Here's how the part is built. I have some questions about the finished solid (model axes, mm). A direction names the side the tool comes from. Give positions to 0.01 mm unless a question says otherwise; leave off trailing zeros. Loops run counter-clockwise (first coordinate to the right, second up) from the corner with the lowest first, then second, coordinate; pieces in that order, holes last. Notation, with made-up numbers: (-18.75, -27) -> (-8.75, -27) arc R22 ccw to (-8.75, -14) -> close; hole circle Ø4 at (10, -3). An arc over 180 degrees is marked (long way). Answer in a Markdown table with one row per item. Add a question column.
Item 1: If I drill on line 1 (Z direction, x = 0, y = -0.5); line 2 (X direction, y = -3.5, z = -223); line 3 (X direction, y = -0.5, z = -308.5), over which ranges is the centre line in solid material (lowest first)?
Item 2: For P1, Ø1.5, axis at x = 2.5, z = -62.5, coming from the +Y side; P2, Ø3.5, axis at x = 0, z = -308.5, coming from the -Y side; P3, Ø3, axis at x = -1, z = -114, coming from the -Y side, each with a flat end and sliding along its axis, tell me the tip position at first contact or that it passes through.
Item 3: If we section it at A-A (y = -8.75): Write out the boundary of the cut face in (x, z), then the cut area to 3 significant figures.
Item 4: Which directions (+Z, -Z, +X, -X, +Y, -Y) give clear straight access to the entire face, cutting with the end or side of a thin tool? Please do faces 1 (the face through (5.016, -7, -175)), 2 (the face through (1, -1, 0)).
Item 5: If we section it at C-C (x = -0.25): Write out the boundary of the cut face in (y, z), then the cut area to 3 significant figures.
Item 6: We'd pull the mould along X, two halves only. Please class faces 3 (the face through (0, 0, -175)), 4 (the face through (0, -1.588, -175)), 5 (the face through (6.604, -6, -175)): released by +X, released by -X, zero draft, split by the parting line, or undercut.
Item 7: If we section it at B-B (z = -218): Write out the boundary of the cut face in (x, y), then the cut area to 4 significant figures.
```python
from build123d import *

# Parameters (mm, degrees)
BOSS_EXTRUDE1_DEPTH  = 355
M4_CLEARANCE_HOLE2_D = 4.5


with BuildPart() as part:
    # Sketch1 → Boss-Extrude1 (new body)
    with BuildSketch(Plane.XY):
        Polygon((-6.604, 0), (6.604, 0), (6.604, -12.7), (5.0165, -12.7), (5.0165, -1.5875), (-5.0165, -1.5875), (-5.0165, -12.7), (-6.604, -12.7), align=None)
    extrude(amount=-BOSS_EXTRUDE1_DEPTH)

    # M4 Clearance Hole2 (through all)
    with Locations(Plane(origin=(0, 0, 0), x_dir=(1, 0, 0), z_dir=(0, 1, 0))):
        with Locations((0, 288.5), (0, 7), (0, 348.5), (0, 308.5), (0, 335)):
            Hole(M4_CLEARANCE_HOLE2_D / 2)


solid = part.part
```
Recorded:
| question | item | result |
|---|---|---|
| 1 | line 1 | z = -355 to -350.75, -346.25 to -337.25, -332.75 to -310.75, -306.25 to -290.75, -286.25 to -9.25, -4.75 to 0 |
| 1 | line 2 | x = -6.6 to -5.02, 5.02 to 6.6 |
| 1 | line 3 | x = -6.6 to -2.25, 2.25 to 6.6 |
| 2 | P1 | stops at y = 0 |
| 2 | P2 | passes through |
| 2 | P3 | stops at y = -1.59 |
| 3 | outline | (-6.6, -355) -> (-5.02, -355) -> (-5.02, 0) -> (-6.6, 0) -> close; (5.02, -355) -> (6.6, -355) -> (6.6, 0) -> (5.02, 0) -> close |
| 3 | area | 1,130 mm^2 |
| 4 | face 1 | +Z, -Z, -Y |
| 4 | face 2 | +Z, +X, -X, +Y, -Y |
| 5 | outline | (-1.59, -355) -> (0, -355) -> (0, -350.74) -> (-1.59, -350.74) -> close; (-1.59, -346.26) -> (0, -346.26) -> (0, -337.24) -> (-1.59, -337.24) -> close; (-1.59, -332.76) -> (0, -332.76) -> (0, -310.74) -> (-1.59, -310.74) -> close; (-1.59, -306.26) -> (0, -306.26) -> (0, -290.74) -> (-1.59, -290.74) -> close; (-1.59, -286.26) -> (0, -286.26) -> (0, -9.24) -> (-1.59, -9.24) -> close; (-1.59, -4.76) -> (0, -4.76) -> (0, 0) -> (-1.59, 0) -> close |
| 5 | area | 528 mm^2 |
| 6 | face 3 | zero draft |
| 6 | face 4 | undercut |
| 6 | face 5 | released by +X |
| 7 | outline | (-6.6, -12.7) -> (-5.02, -12.7) -> (-5.02, -1.59) -> (5.02, -1.59) -> (5.02, -12.7) -> (6.6, -12.7) -> (6.6, 0) -> (-6.6, 0) -> close |
| 7 | area | 56.25 mm^2 |
